For this review, take the finished solid that the model builds, in its own axes (mm). A direction names the side the tool comes from. Coordinates: 2 decimals unless noted, no trailing zeros. Loops run counter-clockwise (first coordinate to the right, second up) from the corner with the lowest first, then second, coordinate; pieces in that order, holes last.
1. Clearance check with flat-ended pins moving along their axes: P1, Ø23.5, axis at x = 302, z = 5298, coming from the +Y side; P2, Ø5, axis at x = 439, z = 5440.5, coming from the +Y side. State where each tip first meets the part, or that it passes through.
2. Take a section at D-D, the plane z = 5553. State the section outline as (x, y) points.
3. Machinability: for faces 1 (the face through (505.82, -1228.56, 5397.42)), 2 (the face through (506, -1238.624, 5300)), 3 (the face through (631.62, -1211.62, 5492.57)), which of the approach directions +Z, -Z, +X, -X, +Y, -Y give a long, thin tool a straight path to every point of the face, cutting with its end or side? Answer none if there is none.
4. Take a section at C-C, the plane z = 5390.5. State the section outline as (x, y) points.
5. Take a section at A-A, the plane x = 392. State the section outline as (y, z) points.
6. To check wall thickness, follow probe 1 along Y at (x, z) = (395.5, 5319); probe 2 along Y at (x, z) = (318.5, 5516). State the ranges of each line that lie inside material, in increasing order.
7. Mouldability with a two-part tool opening along Z and no side actions: class faces 4 (the face through (505.818, -1223.562, 5566.656)), 5 (the face through (389.62, -1211.62, 5492.57)), 6 (the face through (505.818, -1228.134, 5563.915)), 7 (the face through (0, -1218, 5453)) as pulls with the +Z half, pulls with the -Z half, needs draft (parallel to the pull), parting line crosses it, or undercut.
8. Take a section at B-B, the plane x = 663.5. State the section outline as (y, z) points.
```python
from build123d import *

# Parameters (mm, degrees)
BOSS_EXTRUDE1_DEPTH     = 1026
CUT_EXTRUDE1_DEPTH      = 5875.695454102
CUT_EXTRUDE1_DEPTH_BACK = 5875.695454102
SKETCH2_R               = 11


with BuildPart() as part:
    # Sketch1 → Boss-Extrude1 (new body)
    with BuildSketch(Plane(origin=(0, 0, 0), x_dir=(0, 0, -1), z_dir=(1, 0, 0))):
        Polygon((-5649.138897543, -1238.689665232), (-5481.830586551, -1208.005375509), (-5314.923755358, -1238.623896007), (-5285.330586551, -1238.623896007), (-5285.330586551, -1243.623896007), (-5315.330586551, -1243.623896007), (-5481.830586551, -1213.072021383), (-5648.330586551, -1243.623896007), align=None)
    extrude(amount=BOSS_EXTRUDE1_DEPTH)

    # Sketch2 → Cut-Extrude1 (cut, two sides: drawn at the far end of the back side and taken through both)
    with BuildSketch(Plane(origin=(0, 0, 0), x_dir=(1, 0, 0), z_dir=(0, 1, 0)).offset(-CUT_EXTRUDE1_DEPTH_BACK)):
        with Locations((50, -5481.830586551)):
            Circle(SKETCH2_R)
        with Locations((150, -5481.830586551)):
            Circle(SKETCH2_R)
        with Locations((976, -5481.830586551)):
            Circle(SKETCH2_R)
        with Locations((876, -5481.830586551)):
            Circle(SKETCH2_R)
        with Locations((634, -5481.830586551)):
            Circle(SKETCH2_R)
        with Locations((392, -5481.830586551)):
            Circle(SKETCH2_R)
    extrude(amount=CUT_EXTRUDE1_DEPTH + CUT_EXTRUDE1_DEPTH_BACK, mode=Mode.SUBTRACT)


solid = part.part
```
Results list:
1. P1: stops at y = -1238.62
1. P2: stops at y = -1215.13
2. outline: (0, -1226.13) - (1026, -1226.13) - (1026, -1221.06) - (0, -1221.06) - close
3. face 1: +X, -X, -Y
3. face 2: -Z, +X, -X, +Y
3. face 3: +Y, -Y
4. outline: (0, -1229.83) - (1026, -1229.83) - (1026, -1224.76) - (0, -1224.76) - close
5. outline: (-1243.62, 5285.33) - (-1238.62, 5285.33) - (-1238.62, 5314.92) - (-1210.02, 5470.83) - (-1215.09, 5470.83) - (-1243.62, 5315.33) - close; (-1243.62, 5648.33) - (-1215.09, 5492.83) - (-1210.02, 5492.83) - (-1238.69, 5649.14) - close
6. probe 1: y = -1242.95 to -1237.88
6. probe 2: y = -1219.34 to -1214.27
7. face 4: pulls with the +Z half
7. face 5: undercut
7. face 6: undercut
7. face 7: needs draft
8. outline: (-1243.62, 5285.33) - (-1238.62, 5285.33) - (-1238.62, 5314.92) - (-1208.01, 5481.83) - (-1238.69, 5649.14) - (-1243.62, 5648.33) - (-1213.07, 5481.83) - (-1243.62, 5315.33) - close
